Can you work these out from the model? Positions are in its coordinate system, mm. A direction names the side the tool comes from. Round coordinates to 2 decimals unless told otherwise and drop trailing zeros. Loops run counter-clockwise (first coordinate to the right, second up) from the corner with the lowest first, then second, coordinate; pieces in that order, holes last. Notation, with made-up numbers: (32.5, 7.25) -> (68.5, 7.25) arc R16 ccw to (68.5, 22.25) -> close; hole circle Ø7 at (71, 4). An arc over 180 degrees is marked (long way). Answer as a JSON object with one key per item and string values.
```python
from build123d import *

# Parameters (mm, degrees)
SKETCH1_W           = 76.2
SKETCH1_H           = 38.1
BOSS_EXTRUDE1_DEPTH = 5.08
SKETCH2_W           = 5.08
SKETCH2_H           = 5.08
CUT_EXTRUDE1_DEPTH  = 5.08


with BuildPart() as part:
    # Sketch1 → Boss-Extrude1 (new body)
    with BuildSketch(Plane(origin=(0, 0, 0), x_dir=(1, 0, 0), z_dir=(0, 1, 0))):
        with Locations((-0.653142857, 12.627428571)):
            Rectangle(SKETCH1_W, SKETCH1_H)
    extrude(amount=BOSS_EXTRUDE1_DEPTH)

    # Sketch2 → Cut-Extrude1 (cut)
    with BuildSketch(Plane(origin=(0, 5.08, 0), x_dir=(1, 0, 0), z_dir=(0, 1, 0))):
        Polygon((1.886857143, 20.247428571), (-3.193142857, 20.247428571), (-3.193142857, 15.167428571), (-8.273142857, 15.167428571), (-8.273142857, 10.087428571), (-3.193142857, 10.087428571), (-3.193142857, 5.007428571), (1.886857143, 5.007428571), (1.886857143, 10.087428571), (6.966857143, 10.087428571), (6.966857143, 15.167428571), (1.886857143, 15.167428571), align=None)
        with Locations((-36.213142857, 18.977428571)):
            Rectangle(SKETCH2_W, SKETCH2_H)
        with Locations((-36.213142857, 29.137428571)):
            Rectangle(SKETCH2_W, SKETCH2_H)
        with Locations((-36.213142857, -3.882571429)):
            Rectangle(SKETCH2_W, SKETCH2_H)
        with Locations((-36.213142857, 6.277428571)):
            Rectangle(SKETCH2_W, SKETCH2_H)
        with Locations((34.906857143, 6.277428571)):
            Rectangle(SKETCH2_W, SKETCH2_H)
        with Locations((34.906857143, -3.882571429)):
            Rectangle(SKETCH2_W, SKETCH2_H)
        with Locations((34.906857143, 29.137428571)):
            Rectangle(SKETCH2_W, SKETCH2_H)
        with Locations((34.906857143, 18.977428571)):
            Rectangle(SKETCH2_W, SKETCH2_H)
    extrude(amount=-CUT_EXTRUDE1_DEPTH, mode=Mode.SUBTRACT)


solid = part.part
```
Q1. If I drill on L1, parallel to Z at x = 33.5, y = 1.4; L2, parallel to X at y = 3.25, z = -17; L3, parallel to Z at x = -6, y = 4.2, over which ranges is the centre line in solid material (lowest first)? Write a range as [from, to].
Determined:
{"L1": "[-26.6, -21.52], [-16.44, -8.82], [-3.74, 1.34]", "L2": "[-33.67, -3.19], [1.89, 32.37]", "L3": "[-31.68, -15.17], [-10.09, 6.42]"}
Q2. On a 3-axis mill with a long thin cutter (end or side, diameter ignored), from which of +Z, -Z, +X, -X, +Y, -Y can I reach the whole of each face in a straight line? I mean faces 4 (the flat face through (35, 3, -8.817)), 5 (the flat face through (32.367, 3, 4)), 6 (the flat face through (-33.673, 3, -6)), 7 (the flat face through (32.367, 3, -29)), 8 (the flat face through (-3.193, 3, -18)). Say none if no direction works.
Determined:
{"face 4": "+X, +Y, -Y", "face 5": "+Z, +X, +Y, -Y", "face 6": "-X, +Y, -Y", "face 7": "-Z, +X, +Y, -Y", "face 8": "+Y, -Y"}
Q3. I want a section at A-A, the plane x = -4. Write out the boundary of the cut face in (y, z), then the cut area to 3 significant figures.
Determined:
{"outline": "(0, -31.68) -> (5.08, -31.68) -> (5.08, -15.17) -> (0, -15.17) -> close; (0, -10.09) -> (5.08, -10.09) -> (5.08, 6.42) -> (0, 6.42) -> close", "area": "168 mm²"}
Q4. I want a section at B-B, the plane z = 3. Write out the boundary of the cut face in (x, y), then the cut area to 3 significant figures.
Determined:
{"outline": "(-33.67, 0) -> (32.37, 0) -> (32.37, 5.08) -> (-33.67, 5.08) -> close", "area": "335 mm²"}
Q5. I'm going to push flat-ended pins straight in: pin 1 (1.5 mm diameter, centred on y = 3, z = -17, fed in from -X); pin 2 (1.5 mm diameter, centred on y = 3.5, z = -18, fed in from -X); pin 3 (1.5 mm diameter, centred on x = -36.5, y = 2.5, fed in from +Z); pin 4 (2.5 mm diameter, centred on x = 36, y = 2.5, fed in from -Z). Where does each tip first touch, or does it pass through?
Determined:
{"pin 1": "x = -38.75", "pin 2": "x = -33.67", "pin 3": "z = 1.34", "pin 4": "z = -26.6"}
Q6. We'd pull the mould along Z, two halves only. Please class faces 1 (the flat face through (-1, 3, -31.677)), 2 (the flat face through (35, 3, 1.343)), 3 (the flat face through (35, 3, -21.517)): pulls with the +Z half, pulls with the -Z half, needs draft (parallel to the pull), parting line crosses it, or undercut.
Determined:
{"face 1": "pulls with the -Z half", "face 2": "pulls with the +Z half", "face 3": "undercut"}
